Autodesk Inventor part; units mm, degrees
ref_plane "YZ Plane" through (0, 0, 0) normal (1, 0, 0) x (0, 1, 0)
ref_plane "XZ Plane" through (0, 0, 0) normal (0, 1, 0) x (-1, 0, 0)
ref_plane "XY Plane" through (0, 0, 0) normal (0, 0, 1) x (1, 0, 0)
sketch "Sketch6" plane through (0, 0, 0) normal (0, 1, 0) x (-1, 0, 0)
  line L0 (0, 0) -> (-436, 0)
  line L1 (-436, 0) -> (-436, -467)
  line L2 (-436, -467) -> (0, -467)
  line L3 (0, -467) -> (0, 0)
  dimension "d25" = 436
  dimension "d26" = 467
extrude "Extrusion5" add sketch "Sketch6" along normal blind 56
sketch "Sketch7" plane through (436, 0, -467) normal (0, 0, -1) x (-1, 0, 0)
  line L0 (436, 0) -> (0, 0)
  line L1 (218, 0) -> (376, 0)
  line L2 (218, 0) -> (376, 0) construction
  line L3 (376, 0) -> (376, 56)
  line L4 (436, 56) -> (0, 56)
  line L5 (376, 56) -> (60, 56)
  line L6 (376, 56) -> (692, 56) construction
  line L7 (60, 56) -> (60, 0)
  line L8 (60, 0) -> (218, 0)
  line L9 (60, 0) -> (160, 0)
  line L10 (160, 0) -> (160, 56)
  line L11 (376, 0) -> (276, 0)
  line L12 (376, 0) -> (476, 0) construction
  line L13 (276, 0) -> (276, 56)
  dimension "d29" = 158
  dimension "d30" = 0
  dimension "d31" = 316
  dimension "d32" = 180
  dimension "d33" = 100
  dimension "d34" = 100
  dimension "d35" = 180
extrude "Extrusion6" add sketch "Sketch7" along normal blind 100 contours L0 L13 L4 L3 | L0 L7 L4 L10
sketch "Sketch8" plane through (0, 0, -467) normal (-1, 0, 0) x (0, 0, 1)
  arc A0 (-53, 44) -> (-53, 12) centre (-53, 28) ccw
  line L0 (0, 0) -> (-100, 0)
  line L1 (-100, 0) -> (-100, 56)
  arc A1 (-53, 54) -> (-53, 2) centre (-53, 28) ccw
  line L2 (0, 0) -> (-100, 0)
  line L3 (-100, 56) -> (-100, 0)
  line L4 (-100, 0) -> (-100, 56)
  line L5 (0, 56) -> (-100, 56)
  line L6 (-100, 56) -> (0, 56)
  line L7 (-53, 54) -> (0, 54)
  line L8 (-53, 12) -> (-40, 12)
  line L9 (-40, 12) -> (-40, 2)
  line L10 (-40, 2) -> (-53, 2)
  line L11 (-53, 44) -> (0, 44)
  line L12 (467, 0) -> (0, 0)
  line L13 (0, 56) -> (0, 0)
  line L14 (0, 44) -> (0, 54)
  point P0 (467, 56)
  dimension "d30" = 0
  dimension "d32" = 180
  dimension "d35" = 180
  dimension "d38" = 28
  dimension "d39" = 32
  dimension "d40" = 47
  dimension "d45" = 52
  dimension "d50" = 13
extrude "Extrusion8" cut sketch "Sketch8" against normal through all contours L11 L13 L0 L1 L5 L7 A1 L10 L9 L8 A0
sketch "Sketch9" plane through (0, 0, -467) normal (-1, 0, 0) x (0, 0, 1)
  line L0 (467, 0) -> (0, 0)
  line L1 (0, 0) -> (467, 0)
  line L2 (467, 0) -> (467, 18)
  line L3 (467, 18) -> (0, 18)
  line L4 (0, 18) -> (0, 0)
  line L5 (0, 0) -> (0, 56)
  line L6 (467, 0) -> (467, 56)
  line L7 (0, 56) -> (467, 56)
  line L8 (467, 56) -> (467, 54)
  line L9 (467, 54) -> (0, 54)
  line L10 (0, 54) -> (0, 56)
  dimension "d59" = 467
  dimension "d60" = 18
  dimension "d61" = 2
extrude "Extrusion9" cut sketch "Sketch9" against normal through all contours L0 L4 L3 L2 | L9 L5 L7 L6
sketch "Sketch10" plane through (0, 54, 0) normal (0, 1, 0) x (1, 0, 0)
  line L0 (376, 520) -> (376, 467)
  line L1 (436, 467) -> (436, 0)
  line L2 (376, 467) -> (436, 467)
  line L3 (436, 467) -> (436, 0)
  line L4 (436, 0) -> (0, 0)
  line L5 (436, 0) -> (0, 0)
  line L6 (0, 467) -> (60, 467)
  line L7 (0, 0) -> (0, 467)
  line L8 (0, 467) -> (60, 467)
  line L9 (60, 467) -> (60, 452)
  line L10 (60, 452) -> (160, 452)
  line L11 (160, 520) -> (160, 467)
  line L12 (160, 452) -> (160, 467)
  line L13 (276, 467) -> (276, 520)
  line L14 (160, 467) -> (276, 467)
  line L15 (276, 467) -> (276, 452)
  line L16 (276, 452) -> (376, 452)
  line L17 (376, 452) -> (376, 467)
  dimension "d64" = 15
  dimension "d65" = 90
extrude "Extrusion10" cut sketch "Sketch10" against normal blind 21
sketch "Sketch11" plane through (0, 33, 0) normal (0, 1, 0) x (1, 0, 0)
  circle A0 centre (218, 218.5) radius 4.25
  line L0 (0, 0) -> (0, 467)
  line L1 (436, 0) -> (0, 0)
  dimension "d70" = 8.5
  dimension "d71" = 218
  dimension "d72" = 218.5
extrude "Extrusion11" cut sketch "Sketch11" against normal through all
sketch "Sketch12" plane through (0, 33, 0) normal (0, 1, 0) x (1, 0, 0)
  circle A0 centre (218, 218.5) radius 4.25
  circle A1 centre (218, 218.5) radius 120
  circle A2 centre (218, 218.5) radius 15
  line L0 (231.9078, 224.1191) -> (329.2621, 263.4528)
  line L1 (233, 218.5) -> (338, 218.5)
  arc A3 (329.2621, 263.4528) -> (231.9078, 224.1191) centre (280.5849, 243.7859) ccw
  circle A4 centre (218, 218.5) radius 145
  circle A5 centre (320.5305, 115.9695) radius 4.5
  circle A6 centre (320.5305, 321.0305) radius 4.5
  circle A7 centre (115.4695, 321.0305) radius 4.5
  circle A8 centre (115.4695, 115.9695) radius 4.5
  line L2 (320.5305, 115.9695) -> (302.8528, 133.6472)
  line L3 (320.5305, 115.9695) -> (345.5305, 115.9695) construction
  line L4 (222.25, 218.5) -> (233, 218.5)
  line L5 (218, 203.5) -> (218, 150.5)
  line L6 (218, 218.5) -> (281, 218.5) construction
  arc A9 (266, 170.5) -> (238, 198.5) centre (218, 150.5) ccw
  line L7 (302.8528, 133.6472) -> (266, 170.5)
  line L8 (238, 198.5) -> (228.6066, 207.8934)
  line L9 (218, 203.5) -> (218, 214.25)
  line L10 (260.9181, 292.4631) -> (298.382, 307.5995)
  point P0 (0, 0)
  dimension "d81" = 290
  dimension "d76" = 30
  dimension "d77" = 240
  dimension "d82" = 9
  dimension "d87" = 360
  dimension "d90" = 135
  dimension "d91" = 22
  dimension "d92" = 68
  dimension "d95" = 52
extrude "Extrusion12" cut sketch "Sketch12" against normal through all contours L1 A1 L7 A9 L8 A2 | A2 L0 A1 L1 | A3 L0 | A5 A4 L2 | L2 A4 A5 | A3 L10 A1 | A5 A4 | A8 A4 | A4 A8 | A6 A4 | A4 A6 | A7 A4 | A4 A7
sketch "Sketch13" plane through (0, 18, -467) normal (0, -1, 0) x (1, 0, 0)
  arc A0 (179.5346, 284.9654) -> (179.5346, 344.9654) centre (219.5346, 314.9654) ccw
  line L0 (144.5346, 344.9654) -> (244.5346, 344.9654)
  line L1 (244.5346, 344.9654) -> (244.5346, 284.9654)
  line L2 (244.5346, 284.9654) -> (144.5346, 284.9654)
  line L3 (144.5346, 284.9654) -> (144.5346, 344.9654)
  point P0 (0, 467)
  point P1 (266, 296.5)
  point P2 (238, 268.5)
  dimension "d96" = 100
  dimension "d97" = 100
  dimension "d98" = 60
  dimension "d99" = 25
  dimension "d100" = 30
extrude "Extrusion13" cut sketch "Sketch13" against normal blind 13 contours L2 L3 L0 L1
sketch "Sketch14" plane through (0, 31, -467) normal (0, -1, 0) x (1, 0, 0)
  line L0 (144.5346, 284.9654) -> (144.5346, 344.9654)
  line L1 (244.5346, 284.9654) -> (144.5346, 284.9654)
  line L2 (244.5346, 344.9654) -> (244.5346, 284.9654)
  line L3 (144.5346, 344.9654) -> (244.5346, 344.9654)
  circle A0 centre (239.5346, 289.9654) radius 1.75
  circle A1 centre (149.5346, 289.9654) radius 1.75
  circle A2 centre (239.5346, 339.9654) radius 1.75
  circle A3 centre (149.5346, 339.9654) radius 1.75
  line L4 (147.0346, 329.9654) -> (151.0346, 329.9654)
  line L5 (151.0346, 329.9654) -> (151.0346, 304.9654)
  line L6 (151.0346, 304.9654) -> (147.0346, 304.9654)
  line L7 (147.0346, 304.9654) -> (147.0346, 329.9654)
  point P0 (0, 467)
  dimension "d103" = 3.5
  dimension "d104" = 5
  dimension "d105" = 5
  dimension "d108" = 90
  dimension "d111" = 50
  dimension "d117" = 4
  dimension "d118" = 25
  dimension "d119" = 15
  dimension "d120" = 2.5
extrude "Extrusion14" cut sketch "Sketch14" against normal through all contours A0 | A1 | A2 | A3 | L4 L5 L6 L7
chamfer "Chamfer1" distance 1 angle 45 4 edges at (147.7846, 33, -177.0346) (147.7846, 33, -127.0346) (237.7846, 33, -127.0346) (237.7846, 33, -177.0346)
properties part number "bin_lid"
Design review of the part built by this model. Coordinates are the model's own, in mm. A direction names the side the tool comes from. Coordinates: 2 decimals unless noted, no trailing zeros. Write each loop counter-clockwise with the first axis right and the second up, starting at its lowest first coordinate (ties: lowest second). Pieces come first, ordered by that corner, then holes. Notation, with made-up numbers: (9.25, 86) -> (31.25, 86) arc R32 ccw to (31.25, 114) -> close; hole circle Ø9 at (15.5, 38.5). An arc over 180 degrees is marked (long way). Write each question's results on one line, items separated by ' | '. Start each with the question number.
(1) Take a section at C-C on z = -427.5. Write out the cut boundary in (x, y).
(2) The part is to be moulded in two halves that separate along Z. For faces 1 (the face through (325, 28, -536)), 2 (the face through (215, 25, 0)), 3 (the face through (276, 46, -510)), say which applies: pulls with the +Z half, pulls with the -Z half, needs draft (parallel to the pull), parting line crosses it, or undercut.
(3) Take a section at B-B on x = 360. Write out the cut boundary in (y, z).
(4) Clearance check with flat-ended pins moving along their axes: P1, Ø4, axis at x = 149.53, z = -127.03, coming from the -Y side; P2, Ø5.5, axis at x = 115.47, z = -115.97, coming from the -Y side; P3, Ø12, axis at x = 117.5, z = -343, coming from the -Y side; P4, Ø12, axis at x = 268, y = 24, coming from the -Z side. State where each tip first meets the part, or that it passes through.
(5) Take a section at A-A on z = -150. Write out the cut boundary in (x, y).
(6) For line 1 along X through (y, z) = (7, -510.5); line 2 along Y through (x, z) = (355, -209.5); line 3 along Z through (x, y) = (178, 19), list the stretches that pass through material, from the lowest coordinate up. Write a range as from..to.
(7) Tool access review of faces 4 (the face through (221, 28, -467)), 5 (the face through (109, 44, -452)), 6 (the face through (195, 24, -182.035)): name each direction out of +Z, -Z, +X, -X, +Y, -Y from which nothing blocks a thin tool from reaching the whole face with its end or side.
Results found:
1) outline: (0, 18) -> (436, 18) -> (436, 33) -> (0, 33) -> close
2) face 1: undercut | face 2: pulls with the +Z half | face 3: needs draft
3) outline: (2, -520) arc R26 ccw to (54, -520) -> (54, -452) -> (33, -452) -> (33, 0) -> (18, 0) -> (18, -467) -> (44, -467) -> (44, -520) arc R16 cw to (12, -520) -> (12, -507) -> (2, -507) -> close
4) P1: stops at y = 31 | P2: passes through | P3: stops at y = 18 | P4: stops at z = -467
5) outline: (0, 18) -> (144.53, 18) -> (144.53, 31) -> (147.03, 31) -> (147.03, 33) -> (0, 33) -> close; (151.03, 31) -> (244.53, 31) -> (244.53, 18) -> (286.5, 18) -> (286.5, 33) -> (151.03, 33) -> close; (316.53, 18) -> (436, 18) -> (436, 33) -> (316.53, 33) -> close
6) line 1: x = 60..160, 276..376 | line 2: y = 18..33 | line 3: z = -467..-182.03, -122.03..0
7) face 4: +X, -X, -Y | face 5: +Z, +X, -X, +Y | face 6: -Y
